Here's the drawing with two shaded views (mm, measured from the low corner). I have some questions. A direction names the side the tool comes from. Coordinates: 2 decimals unless noted, no trailing zeros. Loops run counter-clockwise (first coordinate to the right, second up) from the corner with the lowest first, then second, coordinate; pieces in that order, holes last. Notation, with made-up numbers: M 23.5,-34 L 48.5,-34 A7 cw 48.5,-24 Z; hole C -12.5,58 d3. An arc over 180 degrees is marked long. Use one line per item in the form item = value. Start each with the question number.
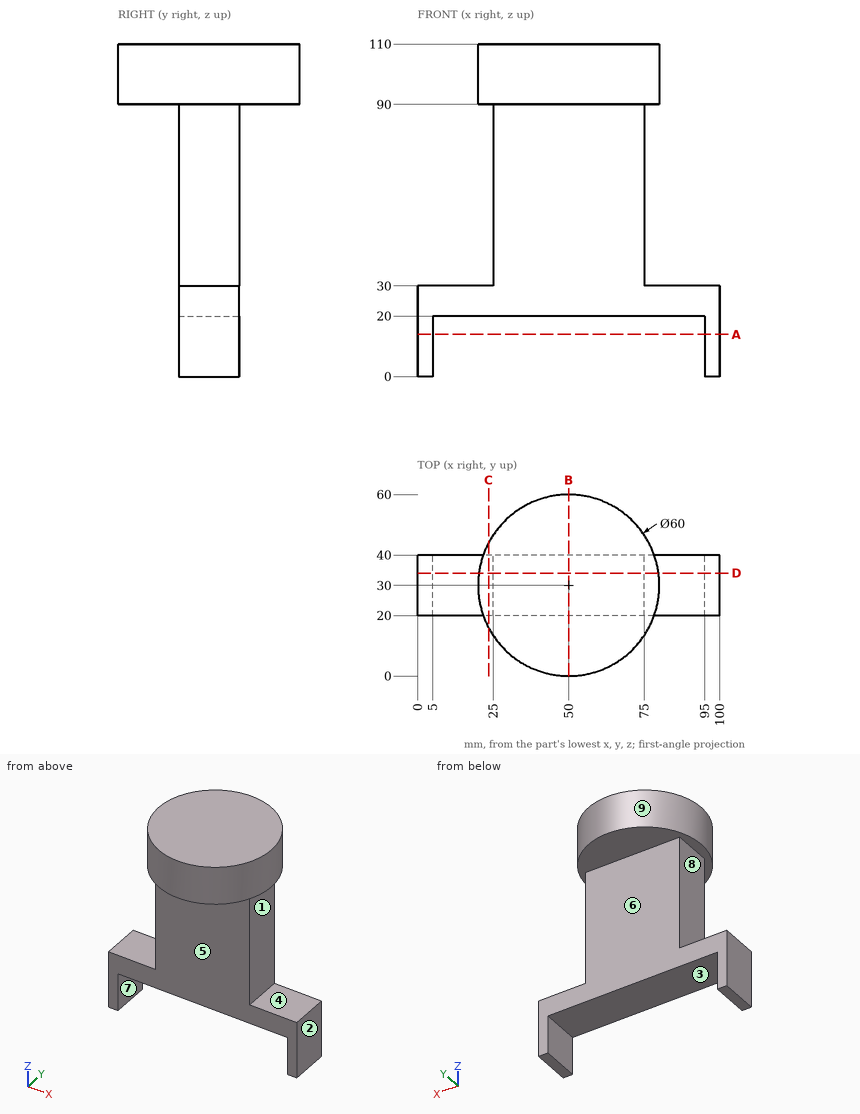
Item 1: I want a section at A-A (z = 14). Write out the boundary of the cut face in (x, y), plus the area to 3 significant figures.
Item 2: I want a section at B-B (x = 50). Write out the boundary of the cut face in (y, z), plus the area to 3 significant figures.
Item 3: Thinking about a two-plate mould opening in Z: for the marked faces 1, 2, 3 and 4, which applies, pulls with the +Z half, pulls with the -Z half, needs draft (parallel to the pull), parting line crosses it, or undercut?
Item 4: I want a section at C-C (x = 23.5). Write out the boundary of the cut face in (y, z).
Item 5: Please list where these lines run through material, in increasing order: line 1 along Z through (x, y) = (21, 25.5); line 2 along Z through (x, y) = (42, 57); line 3 along Y through (x, z) = (56, 33.5).
Item 6: For the marked faces 5, 6, 7, 8 and 9, which set-ups out of +Z, -Z, +X, -X, +Y, -Y let a thin tool reach every point of the face, with its end or its side?
Item 7: I'm going to push flat-ended pins straight in: P1, Ø5, axis at x = 13.5, y = 32.5, coming from the +Z side; P2, Ø2, axis at y = 39, z = 66.5, coming from the -X side; P3, Ø10, axis at y = 52.5, z = 98, coming from the -X side. Where does each tip first touch, or does it pass through?
Item 8: I want a section at D-D (y = 34). Write out the boundary of the cut face in (x, z), plus the area to 3 significant figures.
Worked answers:
q1.outline = M 0,20 L 5,20 L 5,40 L 0,40 Z; M 95,20 L 100,20 L 100,40 L 95,40 Z
q1.area = 200 mm²
q2.outline = M 0,90 L 20,90 L 20,20 L 40,20 L 40,90 L 60,90 L 60,110 L 0,110 Z
q2.area = 2,600 mm²
q3.face_1 = undercut
q3.face_2 = needs draft
q3.face_3 = pulls with the -Z half
q3.face_4 = undercut
q4.outline = M 15.94,90 L 44.06,90 L 44.06,110 L 15.94,110 Z; M 20,20 L 40,20 L 40,30 L 20,30 Z
q5.line_1 = 20 to 30, 90 to 110
q5.line_2 = 90 to 110
q5.line_3 = 20 to 40
q6.face_5 = -Z, +X, -X, -Y
q6.face_6 = -Z, +X, -X, +Y
q6.face_7 = -Z, +Y, -Y
q6.face_8 = -X, +Y, -Y
q6.face_9 = +Z
q7.P1 = 30
q7.P2 = 25
q7.P3 = 25.63
q8.outline = M 0,0 L 5,0 L 5,20 L 95,20 L 95,0 L 100,0 L 100,30 L 75,30 L 75,90 L 79.73,90 L 79.73,110 L 20.27,110 L 20.27,90 L 25,90 L 25,30 L 0,30 Z
q8.area = 5,390 mm²
